from build123d import *

# Parameters (mm, degrees)
F0_R     = 63.5
F1_DEPTH = 25.4
F2_W     = 50.8
F2_H     = 25.4
F3_DEPTH = 25.401


with BuildPart() as f1:
    # F0 (on Top) → F1 (new body)
    with BuildSketch(Plane.XY):
        Circle(F0_R)
    extrude(amount=-F1_DEPTH)

    # F2 (on face) → F3 (cut, through all)
    with BuildSketch(Plane.XY):
        Rectangle(F2_W, F2_H)
    extrude(amount=-F3_DEPTH, mode=Mode.SUBTRACT)


solid = f1.part
Work out the finished part from the listing and answer in its coordinate system (mm). A direction names the side the tool comes from. Round coordinates to 2 decimals unless told otherwise and drop trailing zeros. Order: outer loops, then holes, each group sorted by start corner. A loop starts at its lowest first (then second) coordinate and runs counter-clockwise, first axis right, second up. Notation, with made-up numbers: M -30.75,-3 L 14.25,-3 A20 cw 14.25,30 Z; hole C 39.25,-34.5 d2. An arc over 180 degrees is marked long. One line per item, written item: value.
Q1. Determine the mould class of faces 3 (the face through (-1, -13, 0)), 4 (the face through (0, -12.7, -13)), 5 (the face through (-13.77, -61.99, -12.52)) for opening direction X: released by +X, released by -X, zero draft, split by the parting line, or undercut.
Derived:
face 3: zero draft
face 4: undercut
face 5: split by the parting line
Q2. Find section C-C on z = -12.5. Write down the section's boundary in (x, y).
Derived:
outline: C 0,0 d127; hole M -25.4,-12.7 L 25.4,-12.7 L 25.4,12.7 L -25.4,12.7 Z
Q3. Find section B-B on x = 0. Write down the section's boundary in (y, z), then the cut area to 3 significant figures.
Derived:
outline: M -63.5,-25.4 L -12.7,-25.4 L -12.7,0 L -63.5,0 Z; M 12.7,-25.4 L 63.5,-25.4 L 63.5,0 L 12.7,0 Z
area: 2,580 mm²
Q4. For faces 1 (the face through (-1, -13, -25.4)), 2 (the face through (0, 12.7, -13)), determine the directions among +Z, -Z, +X, -X, +Y, -Y from which every point of the face is accessible in a straight line to the end or side of a thin tool.
Derived:
face 1: -Z, +X, -X, +Y, -Y
face 2: +Z, -Z
Q5. Find section A-A on y = 0. Write down the section's boundary in (x, z).
Derived:
outline: M -63.5,-25.4 L -25.4,-25.4 L -25.4,0 L -63.5,0 Z; M 25.4,-25.4 L 63.5,-25.4 L 63.5,0 L 25.4,0 Z
Q6. Find section D-D on y = 56.5. Write down the section's boundary in (x, z).
Derived:
outline: M -28.98,-25.4 L 28.98,-25.4 L 28.98,0 L -28.98,0 Z
Q7. Flat-ended cylindrical pins translate along their axes: pin 1 (2 mm diameter, centred on x = -13.5, z = -5.5, fed in from -Y); pin 2 (3 mm diameter, centred on x = 26, z = -20.5, fed in from +Y); pin 3 (10 mm diameter, centred on x = 9.5, z = -15.5, fed in from +Y). Find the tip coordinate at first contact, or state that the pin passes through.
Derived:
pin 1: y = -62.26
pin 2: y = 58.58
pin 3: y = 63.34
Q8. Straight lines are drawn through the part: line 1 (Y direction, x = -1, z = -4.25); line 2 (X direction, y = 6, z = -17.5); line 3 (Y direction, x = 14, z = -5). For each, find the intervals that lie inside material, in ascending order.
Derived:
line 1: -63.49 to -12.7, 12.7 to 63.49
line 2: -63.22 to -25.4, 25.4 to 63.22
line 3: -61.94 to -12.7, 12.7 to 61.94
